from build123d import *

# Parameters (mm, degrees)
SKETCH1_W                = 71
SKETCH1_H                = 13.8
SKETCH1_W_2              = 67
SKETCH1_H_2              = 9.8
EXTRUDE_THIN1_DEPTH      = 69.85
BOSS_EXTRUDE2_DEPTH      = 11.55
BOSS_EXTRUDE2_DEPTH_BACK = 2.25
SKETCH5_W                = 71
SKETCH5_H                = 8
SKETCH6_W                = 12.7
SKETCH6_H                = 9.856323991
CUT_EXTRUDE1_DEPTH       = 6.8


with BuildPart() as part:
    # Sketch1 → Extrude-Thin1 (new body)
    with BuildSketch(Plane.XY):
        with Locations((33.25, 4.65)):
            Rectangle(SKETCH1_W, SKETCH1_H)
        with Locations((33.25, 4.65)):
            Rectangle(SKETCH1_W_2, SKETCH1_H_2, mode=Mode.SUBTRACT)
    extrude(amount=EXTRUDE_THIN1_DEPTH)

    # Sketch5 → Boss-Extrude2 (add, two sides: drawn at the far end of the back side and taken through both)
    with BuildSketch(Plane(origin=(0, 0, 0), x_dir=(1, 0, 0), z_dir=(0, 1, 0)).offset(-BOSS_EXTRUDE2_DEPTH_BACK)):
        with Locations((33.25, 4)):
            Rectangle(SKETCH5_W, SKETCH5_H)
    extrude(amount=BOSS_EXTRUDE2_DEPTH + BOSS_EXTRUDE2_DEPTH_BACK)

    # Sketch6 → Cut-Extrude1 (cut)
    with BuildSketch(Plane.XY):
        with Locations((13.18, 6.988161996)):
            Rectangle(SKETCH6_W, SKETCH6_H)
    extrude(amount=-CUT_EXTRUDE1_DEPTH, mode=Mode.SUBTRACT)


solid = part.part
Input: part model. Units: mm. Frame: model coordinates. A direction names the side the tool comes from. Round coordinates to 2 decimals unless told otherwise and drop trailing zeros. Order: outer loops, then holes, each group sorted by start corner. A loop starts at its lowest first (then second) coordinate and runs counter-clockwise, first axis right, second up.
1. Pin query (flat end, axial travel): P1, Ø3, axis at x = 14.5, y = 5, coming from the +Z side; P2, Ø3, axis at x = 38.5, y = 4.5, coming from the +Z side. Return the tip coordinate at first contact, or that it passes through.
The answers:
P1: stops at z = -6.8
P2: stops at z = 0
2. Material intervals for line 1 (X direction, y = 5, z = 66.5); line 2 (Y direction, x = 38.5, z = 4.5); line 3 (Z direction, x = 16.5, y = 10.5), sorted ascending.
The answers:
line 1: x = -2.25 to -0.25, 66.75 to 68.75
line 2: y = -2.25 to -0.25, 9.55 to 11.55
line 3: z = -8 to -6.8, 0 to 69.85
3. Mould query, pull axis Y, two halves, no side actions, for faces 4 (the face through (33, 10, 69.85)), 5 (the face through (13, 2.06, -3)), 6 (the face through (66.75, 5, 34)), 7 (the face through (33, -2.25, 30)). Classes: released by +Y, released by -Y, zero draft, split by the parting line, or undercut.
The answers:
face 4: zero draft
face 5: released by +Y
face 6: undercut
face 7: released by -Y
4. Set-up query: faces 1 (the face through (68.75, 5, 31)), 2 (the face through (-0.25, 5, 34)), 3 (the face through (13, 7, -6.8)). Return all of +Z, -Z, +X, -X, +Y, -Y with unobstructed straight access to the full face (end or side cutting, diameter ignored); none if empty.
The answers:
face 1: +Z, -Z, +X, +Y, -Y
face 2: +Z
face 3: +Y
5. Cut plane C-C, the plane x = 3. Output: boundary loops of the cut face in (y, z).
The answers:
outline: (-2.25, -8) - (11.55, -8) - (11.55, 69.85) - (9.55, 69.85) - (9.55, 0) - (-0.25, 0) - (-0.25, 69.85) - (-2.25, 69.85) - close
6. Cut plane A-A, the plane z = 9. Output: boundary loops of the cut face in (x, y).
The answers:
outline: (-2.25, -2.25) - (68.75, -2.25) - (68.75, 11.55) - (-2.25, 11.55) - close; hole (-0.25, -0.25) - (66.75, -0.25) - (66.75, 9.55) - (-0.25, 9.55) - close
7. Cut plane B-B, the plane y = 4. Output: boundary loops of the cut face in (x, z).
The answers:
outline: (-2.25, -8) - (68.75, -8) - (68.75, 69.85) - (66.75, 69.85) - (66.75, 0) - (19.53, 0) - (19.53, -6.8) - (6.83, -6.8) - (6.83, 0) - (-0.25, 0) - (-0.25, 69.85) - (-2.25, 69.85) - close
